Read the model definition and answer for the solid it produces. Units are mm, in the model's axes. Give positions to 0.01 mm unless a question says otherwise; leave off trailing zeros. Loops run counter-clockwise (first coordinate to the right, second up) from the corner with the lowest first, then second, coordinate; pieces in that order, holes last. Notation, with made-up numbers: (-10.5, 20.5) - (18.5, 20.5) arc R28 ccw to (18.5, 47.5) - close; hole circle Ø7 at (-0.75, -11.5). An arc over 180 degrees is marked (long way). Put each result on its own line as item: value. Start each with the question number.
1. Consider L1, parallel to Y at x = 5, z = -12.75. Determine where the line is inside the solid, lowest interval first. Write a range as from..to.
2. Given pin 1 Ø0.8 at (y, z) = (17, -14.5) entering from +X; pin 2 Ø0.8 at (x, y) = (1.5, 17) entering from -Z; pin 3 Ø0.5 at (x, y) = (1.5, 16) entering from +Z, each flat-ended and moving along its own axis, determine where each tip first touches the part or whether it passes through.
3. A cutting plane is placed at A-A, the plane y = 17. Determine the outline of the cut face in (x, z).
4. A cutting plane is placed at B-B, the plane z = -14.25. Determine the outline of the cut face in (x, y), plus the area to 3 significant figures.
5. A cutting plane is placed at C-C, the plane x = 3.75. Determine the outline of the cut face in (y, z).
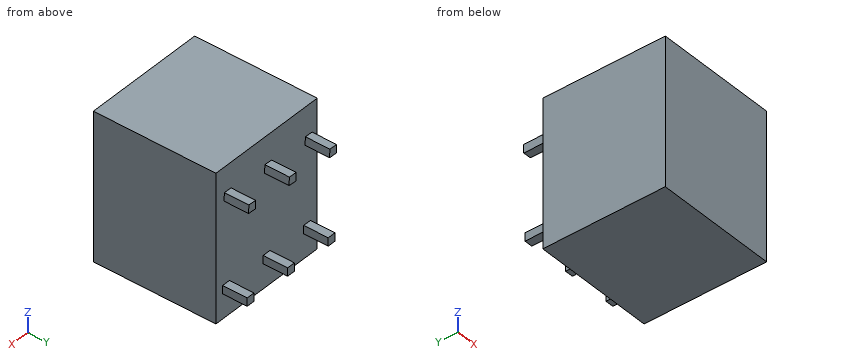
```python
from build123d import *

# Parameters (mm, degrees)
ESQUISSE1_W        = 15
ESQUISSE1_H        = 18
BOSS_EXTRU_1_DEPTH = 15
ESQUISSE2_W        = 1
ESQUISSE2_H        = 1
BOSS_EXTRU_2_DEPTH = 3


with BuildPart() as part:
    # Esquisse1 → Boss.-Extru.1 (new body)
    with BuildSketch(Plane(origin=(0, 0, 0), x_dir=(1, 0, 0), z_dir=(0, 1, 0))):
        with Locations((7.5, 9)):
            Rectangle(ESQUISSE1_W, ESQUISSE1_H)
    extrude(amount=BOSS_EXTRU_1_DEPTH)

    # Esquisse2 → Boss.-Extru.2 (add)
    with BuildSketch(Plane(origin=(0, 15, 0), x_dir=(1, 0, 0), z_dir=(0, 1, 0))):
        with Locations((1.5, 14.5)):
            Rectangle(ESQUISSE2_W, ESQUISSE2_H)
        with Locations((7.5, 14.5)):
            Rectangle(ESQUISSE2_W, ESQUISSE2_H)
        with Locations((13.5, 14.5)):
            Rectangle(ESQUISSE2_W, ESQUISSE2_H)
        Polygon((12.746406665, 3.090573879), (12.788974359, 4.089667464), (13.788067944, 4.04709977), (13.745500249, 3.048006185), align=None)
        Polygon((7.75093874, 3.30341235), (7.793506434, 4.302505935), (6.794412849, 4.34507363), (6.751845155, 3.345980045), align=None)
        Polygon((1.756377231, 3.558818516), (1.798944925, 4.557912101), (0.79985134, 4.600479795), (0.757283646, 3.60138621), align=None)
    extrude(amount=BOSS_EXTRU_2_DEPTH)


solid = part.part
```
Return value:
1. L1: y = 0..15
2. pin 1: stops at x = 14
2. pin 2: stops at z = -15
2. pin 3: stops at z = -3.56
3. outline: (0.76, -3.6) - (0.8, -4.6) - (1.8, -4.56) - (1.76, -3.56) - close; (1, -15) - (2, -15) - (2, -14) - (1, -14) - close; (6.75, -3.35) - (6.79, -4.35) - (7.79, -4.3) - (7.75, -3.3) - close; (7, -15) - (8, -15) - (8, -14) - (7, -14) - close; (12.75, -3.09) - (12.79, -4.09) - (13.79, -4.05) - (13.75, -3.05) - close; (13, -15) - (14, -15) - (14, -14) - (13, -14) - close
4. outline: (0, 0) - (15, 0) - (15, 15) - (14, 15) - (14, 18) - (13, 18) - (13, 15) - (8, 15) - (8, 18) - (7, 18) - (7, 15) - (2, 15) - (2, 18) - (1, 18) - (1, 15) - (0, 15) - close
4. area: 234 mm2
5. outline: (0, -18) - (15, -18) - (15, 0) - (0, 0) - close
